from build123d import *

# Parameters (mm, degrees)
F0_R     = 138.5
F0_R_2   = 108.5
F1_DEPTH = 100
F3_DEPTH = 25
F5_DEPTH = 25


with BuildPart() as f1:
    # F0 (on Top) → F1 (new body)
    with BuildSketch(Plane.XY):
        Circle(F0_R)
        Circle(F0_R_2, mode=Mode.SUBTRACT)
    extrude(amount=F1_DEPTH)

    # F2 (on face) → F3 (cut)
    with BuildSketch(Plane.XY.offset(100)):
        with BuildLine():
            ThreePointArc((-2.499860907, 118.473628692), (0, 118.5), (2.499860907, 118.473628692))
            ThreePointArc((2.499860907, 118.473628692), (2.4999652265, 118.4868141626), (2.5, 118.5))
            ThreePointArc((2.5, 118.5), (-0.0131858374, 120.9999652265), (-2.499860907, 118.473628692))
        make_face()
        with BuildLine():
            ThreePointArc((-2.499860907, 118.473628692), (0, 116), (2.499860907, 118.473628692))
            ThreePointArc((2.499860907, 118.473628692), (0, 118.5), (-2.499860907, 118.473628692))
        make_face()
        with BuildLine():
            ThreePointArc((-116, 0), (-116.7229338406, 1.7584185693), (-118.473628692, 2.499860907))
            ThreePointArc((-118.473628692, 2.499860907), (-118.5, 0), (-118.473628692, -2.499860907))
            ThreePointArc((-118.473628692, -2.499860907), (-116.7229338406, -1.7584185693), (-116, 0))
        make_face()
        with BuildLine():
            ThreePointArc((-118.473628692, -2.499860907), (-118.5, 0), (-118.473628692, 2.499860907))
            ThreePointArc((-118.473628692, 2.499860907), (-121, 0), (-118.473628692, -2.499860907))
        make_face()
        with BuildLine():
            ThreePointArc((118.473628692, -2.499860907), (118.4934069896, -1.25), (118.5, 0))
            ThreePointArc((118.5, 0), (118.4934069896, 1.25), (118.473628692, 2.499860907))
            ThreePointArc((118.473628692, 2.499860907), (116, 0), (118.473628692, -2.499860907))
        make_face()
        with BuildLine():
            ThreePointArc((118.473628692, 2.499860907), (118.4934069896, 1.25), (118.5, 0))
            ThreePointArc((118.5, 0), (118.4934069896, -1.25), (118.473628692, -2.499860907))
            ThreePointArc((118.473628692, -2.499860907), (120.2584185693, -1.7770661594), (121, 0))
            ThreePointArc((121, 0), (120.2584185693, 1.7770661594), (118.473628692, 2.499860907))
        make_face()
        with BuildLine():
            ThreePointArc((-2.499860907, -118.473628692), (0, -118.5), (2.499860907, -118.473628692))
            ThreePointArc((2.499860907, -118.473628692), (0, -116), (-2.499860907, -118.473628692))
        make_face()
        with BuildLine():
            ThreePointArc((2.5, -118.5), (2.4999652265, -118.4868141626), (2.499860907, -118.473628692))
            ThreePointArc((2.499860907, -118.473628692), (0, -118.5), (-2.499860907, -118.473628692))
            ThreePointArc((-2.499860907, -118.473628692), (-0.0131858374, -120.9999652265), (2.5, -118.5))
        make_face()
    extrude(amount=-F3_DEPTH, mode=Mode.SUBTRACT)

    # F4 (on face) → F5 (cut)
    with BuildSketch(Plane(origin=(0, 0, 0), x_dir=(1, 0, 0), z_dir=(0, 0, -1))):
        with BuildLine():
            ThreePointArc((-2.499860907, 118.473628692), (0, 118.5), (2.499860907, 118.473628692))
            ThreePointArc((2.499860907, 118.473628692), (2.4999652265, 118.4868141626), (2.5, 118.5))
            ThreePointArc((2.5, 118.5), (-0.0131858374, 120.9999652265), (-2.499860907, 118.473628692))
        make_face()
        with BuildLine():
            ThreePointArc((-2.499860907, 118.473628692), (0, 116), (2.499860907, 118.473628692))
            ThreePointArc((2.499860907, 118.473628692), (0, 118.5), (-2.499860907, 118.473628692))
        make_face()
        with BuildLine():
            ThreePointArc((-118.473628692, -2.499860907), (-118.5, 0), (-118.473628692, 2.499860907))
            ThreePointArc((-118.473628692, 2.499860907), (-121, 0), (-118.473628692, -2.499860907))
        make_face()
        with BuildLine():
            ThreePointArc((-116, 0), (-116.7229338406, 1.7584185693), (-118.473628692, 2.499860907))
            ThreePointArc((-118.473628692, 2.499860907), (-118.5, 0), (-118.473628692, -2.499860907))
            ThreePointArc((-118.473628692, -2.499860907), (-116.7229338406, -1.7584185693), (-116, 0))
        make_face()
        with BuildLine():
            ThreePointArc((118.473628692, -2.499860907), (118.4934069896, -1.25), (118.5, 0))
            ThreePointArc((118.5, 0), (118.4934069896, 1.25), (118.473628692, 2.499860907))
            ThreePointArc((118.473628692, 2.499860907), (116, 0), (118.473628692, -2.499860907))
        make_face()
        with BuildLine():
            ThreePointArc((118.473628692, 2.499860907), (118.4934069896, 1.25), (118.5, 0))
            ThreePointArc((118.5, 0), (118.4934069896, -1.25), (118.473628692, -2.499860907))
            ThreePointArc((118.473628692, -2.499860907), (120.2584185693, -1.7770661594), (121, 0))
            ThreePointArc((121, 0), (120.2584185693, 1.7770661594), (118.473628692, 2.499860907))
        make_face()
        with BuildLine():
            ThreePointArc((-2.499860907, -118.473628692), (0, -118.5), (2.499860907, -118.473628692))
            ThreePointArc((2.499860907, -118.473628692), (0, -116), (-2.499860907, -118.473628692))
        make_face()
        with BuildLine():
            ThreePointArc((2.5, -118.5), (2.4999652265, -118.4868141626), (2.499860907, -118.473628692))
            ThreePointArc((2.499860907, -118.473628692), (0, -118.5), (-2.499860907, -118.473628692))
            ThreePointArc((-2.499860907, -118.473628692), (-0.0131858374, -120.9999652265), (2.5, -118.5))
        make_face()
    extrude(amount=-F5_DEPTH, mode=Mode.SUBTRACT)


solid = f1.part
Read the model definition and answer for the solid it produces. Units are mm, in the model's axes. Coordinates: 2 decimals unless noted, no trailing zeros. Write each loop counter-clockwise with the first axis right and the second up, starting at its lowest first coordinate (ties: lowest second). Pieces come first, ordered by that corner, then holes. Notation, with made-up numbers: (74.5, -5.5) -> (87.5, -5.5) arc R27 cw to (87.5, 19.5) -> close; hole circle Ø2 at (12.5, 20). An arc over 180 degrees is marked (long way). Return JSON: item names as keys, results as strings.
(1) The part is cut by section C-C on y = -59.5. Give the vertices of the cut face in (x, z), then the cut area to 3 significant figures.
Answers below:
{"outline": "(-125.07, 0) -> (-90.73, 0) -> (-90.73, 100) -> (-125.07, 100) -> close; (90.73, 0) -> (125.07, 0) -> (125.07, 100) -> (90.73, 100) -> close", "area": "6,870 mm^2"}
(2) For a pull along Y with two mould halves and no side action, classify faces 1 (the cylindrical face through (103.49, 32.59, 49.3)), 2 (the cylindrical face through (-18.03, 137.32, 49.3)), 3 (the flat face through (-83, -71, 0)) as pulls with the +Y half, pulls with the -Y half, needs draft (parallel to the pull), parting line crosses it, or undercut.
Answers below:
{"face 1": "undercut", "face 2": "parting line crosses it", "face 3": "needs draft"}
(3) Consider line 1 along Y through (x, z) = (0, 49); line 2 along X through (y, z) = (3.5, 69); line 3 along Y through (x, z) = (48, 21). Determine where each line is inside the solid, lowest interval first. Write a range as from..to.
Answers below:
{"line 1": "-138.5..-108.5, 108.5..138.5", "line 2": "-138.46..-108.44, 108.44..138.46", "line 3": "-129.92..-97.3, 97.3..129.92"}
(4) Each of these flat-tipped pins is pushed along its axis until it touches: P1, Ø8, axis at x = -57.5, z = 83.5, coming from the -Y side; P2, Ø1, axis at y = 97, z = 73.5, coming from the +X side; P3, Ø12, axis at x = 96, z = 47, coming from the +Y side. Where does it stop, or does it pass through?
Answers below:
{"P1": "y = -127.75", "P2": "x = 99.35", "P3": "y = 105.27"}
(5) The part is cut by section D-D on z = 68. Give the vertices of the cut face in (x, y), then the cut area to 3 significant figures.
Answers below:
{"outline": "circle Ø277 at (0, 0); hole circle Ø217 at (0, 0)", "area": "23,300 mm^2"}
(6) The part is cut by section A-A on x = 75. Give the vertices of the cut face in (y, z).
Answers below:
{"outline": "(-116.44, 0) -> (-78.4, 0) -> (-78.4, 100) -> (-116.44, 100) -> close; (78.4, 0) -> (116.44, 0) -> (116.44, 100) -> (78.4, 100) -> close"}
(7) The part is cut by section B-B on z = 88.5. State how many separate pieces and enclosed holes the cut face has, then the cut area to 3 significant figures.
Answers below:
{"separate pieces": "1", "enclosed holes": "5", "area": "23,200 mm^2"}
